Source: CAD feature listing. Evaluate the final solid. Frame: model axes, mm. Face numbers are marked on the shaded views. A direction names the side the tool comes from. Give positions to 0.01 mm unless a question says otherwise; leave off trailing zeros. Loops run counter-clockwise (first coordinate to the right, second up) from the corner with the lowest first, then second, coordinate; pieces in that order, holes last. Notation, with made-up numbers: M -25,39 L 30,39 A23 ccw 30,78 Z; hole C 64.25,-8.75 d1. An arc over 180 degrees is marked long. Answer in a Markdown table with one row per item.
```python
from build123d import *

# Parameters (mm, degrees)
BOSS_EXTRUDE1_DEPTH           = 12.7
SKETCH3_W                     = 9.525
SKETCH3_H                     = 3.683
BOSS_EXTRUDE2_DEPTH           = 1.2573
BOSS_EXTRUDE2_DRAFT           = 24.44
BOSS_EXTRUDE2_PROFILE_2_DEPTH = 1.2573
BOSS_EXTRUDE2_PROFILE_2_DRAFT = 24.44
BOSS_EXTRUDE2_PROFILE_3_DEPTH = 1.2573
BOSS_EXTRUDE2_PROFILE_3_DRAFT = 24.44
SKETCH2_W                     = 1.5875
SKETCH2_H                     = 4.191
BOSS_EXTRUDE3_DEPTH           = 5.3848
SKETCH4_W                     = 3.96875
SKETCH4_H                     = 4.191
BOSS_EXTRUDE4_DEPTH           = 3.175
CUT_EXTRUDE1_START            = -14.351
CUT_EXTRUDE1_DEPTH            = 14.351
FILLET1_R                     = 0.254


with BuildPart() as part:
    # Sketch1 → Boss-Extrude1 (new body)
    with BuildSketch(Plane.XY):
        with BuildLine():
            Line((3.554693097, 0.436578304), (13.826745412, 12.247578304))
            ThreePointArc((13.826745412, 12.247578304), (14.024174489, 13.607523715), (12.868461386, 14.351))
            Line((12.868461386, 14.351), (0, 14.351))
            Line((0, 14.351), (0, 0))
            Line((0, 0), (2.596409071, 0))
            ThreePointArc((2.596409071, 0), (3.122932786, 0.114286897), (3.554693097, 0.436578304))
        make_face()
    extrude(amount=BOSS_EXTRUDE1_DEPTH)


with BuildPart() as boss_extrude2_tool:
    # Sketch3 → Boss-Extrude2 (with draft: the straight prism first)
    with BuildSketch(Plane.ZY):
        with Locations((6.35, 7.1755)):
            Rectangle(SKETCH3_W, SKETCH3_H)
    extrude(amount=BOSS_EXTRUDE2_DEPTH)
    # Boss-Extrude2: the draft: its side faces are tilted about the plane it starts from
    boss_extrude2_sides = [boss_extrude2_tool.faces().sort_by_distance(p)[0] for p in [
        (-0.62865, 7.1755, 1.5875),
        (-0.62865, 5.334, 6.35),
        (-0.62865, 7.1755, 11.1125),
        (-0.62865, 9.017, 6.35),
    ]]
    draft(boss_extrude2_sides, Plane.ZY, BOSS_EXTRUDE2_DRAFT)


with BuildPart() as part_1:
    add(part.part)

    # Boss-Extrude2: add boss_extrude2_tool
    add(boss_extrude2_tool.part)


with BuildPart() as boss_extrude2_profile_2_tool:
    # Sketch3 → Boss-Extrude2 profile 2 (with draft: the straight prism first)
    with BuildSketch(Plane.ZY):
        with Locations((6.35, 12.5095)):
            Rectangle(SKETCH3_W, SKETCH3_H)
    extrude(amount=BOSS_EXTRUDE2_PROFILE_2_DEPTH)
    # Boss-Extrude2 profile 2: the draft: its side faces are tilted about the plane it starts from
    boss_extrude2_profile_2_sides = [boss_extrude2_profile_2_tool.faces().sort_by_distance(p)[0] for p in [
        (-0.62865, 12.5095, 1.5875),
        (-0.62865, 10.668, 6.35),
        (-0.62865, 12.5095, 11.1125),
        (-0.62865, 14.351, 6.35),
    ]]
    draft(boss_extrude2_profile_2_sides, Plane.ZY, BOSS_EXTRUDE2_PROFILE_2_DRAFT)


with BuildPart() as part_2:
    add(part_1.part)

    # Boss-Extrude2 profile 2: add boss_extrude2_profile_2_tool
    add(boss_extrude2_profile_2_tool.part)


with BuildPart() as boss_extrude2_profile_3_tool:
    # Sketch3 → Boss-Extrude2 profile 3 (with draft: the straight prism first)
    with BuildSketch(Plane.ZY):
        with Locations((6.35, 1.8415)):
            Rectangle(SKETCH3_W, SKETCH3_H)
    extrude(amount=BOSS_EXTRUDE2_PROFILE_3_DEPTH)
    # Boss-Extrude2 profile 3: the draft: its side faces are tilted about the plane it starts from
    boss_extrude2_profile_3_sides = [boss_extrude2_profile_3_tool.faces().sort_by_distance(p)[0] for p in [
        (-0.62865, 1.8415, 1.5875),
        (-0.62865, 0, 6.35),
        (-0.62865, 1.8415, 11.1125),
        (-0.62865, 3.683, 6.35),
    ]]
    draft(boss_extrude2_profile_3_sides, Plane.ZY, BOSS_EXTRUDE2_PROFILE_3_DRAFT)


with BuildPart() as part_3:
    add(part_2.part)

    # Boss-Extrude2 profile 3: add boss_extrude2_profile_3_tool
    add(boss_extrude2_profile_3_tool.part)

    # Sketch2 → Boss-Extrude3 (add)
    with BuildSketch(Plane.ZY):
        with Locations((0.79375, 12.2555)):
            Rectangle(SKETCH2_W, SKETCH2_H)
        with Locations((0.79375, 2.0955)):
            Rectangle(SKETCH2_W, SKETCH2_H)
        with Locations((11.90625, 2.0955)):
            Rectangle(SKETCH2_W, SKETCH2_H)
        with Locations((11.90625, 12.2555)):
            Rectangle(SKETCH2_W, SKETCH2_H)
    extrude(amount=BOSS_EXTRUDE3_DEPTH)

    # Sketch4 → Boss-Extrude4 (add)
    with BuildSketch(Plane.ZY.offset(5.3848)):
        with Locations((1.984375, 12.2555)):
            Rectangle(SKETCH4_W, SKETCH4_H)
        with Locations((10.715625, 12.2555)):
            Rectangle(SKETCH4_W, SKETCH4_H)
        with Locations((10.715625, 2.0955)):
            Rectangle(SKETCH4_W, SKETCH4_H)
        with Locations((1.984375, 2.0955)):
            Rectangle(SKETCH4_W, SKETCH4_H)
    extrude(amount=BOSS_EXTRUDE4_DEPTH)

    # Sketch5 → Cut-Extrude1 (cut)
    with BuildSketch(Plane.XZ.offset(CUT_EXTRUDE1_START)):
        Polygon((-5.3848, 3.96875), (-8.5598, 0), (-8.5598, 3.96875), align=None)
        Polygon((-8.5598, 12.7), (-8.5598, 8.73125), (-5.3848, 8.73125), align=None)
    extrude(amount=CUT_EXTRUDE1_DEPTH, mode=Mode.SUBTRACT)

    # Fillet1
    fillet1_edges = [part_3.edges().sort_by_distance(p)[0] for p in [
        (-8.5598, 12.2555, 0),
        (-8.5598, 2.0955, 12.7),
        (-8.5598, 12.2555, 12.7),
        (-8.5598, 2.0955, 0),
    ]]
    fillet(fillet1_edges, radius=FILLET1_R)


solid = part_3.part
```
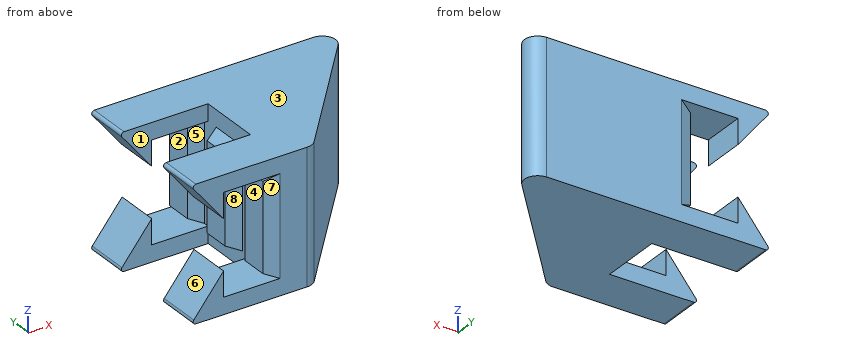
Q1. Contact query for flat-ended pins moving along their axis: pin 1 Ø1.3 at (y, z) = (1.5, 5) entering from -X; pin 2 Ø4 at (x, z) = (10, 3.5) entering from -Y; pin 3 Ø2 at (x, y) = (9, 4) entering from +Z; pin 4 Ø2 at (y, z) = (12.5, 4.5) entering from -X. Output: stop coordinate, or through.
Values follow:
| item | result |
|---|---|
| pin 1 | x = -1.26 |
| pin 2 | y = 5.55 |
| pin 3 | through |
| pin 4 | x = -5.76 |
Q2. Mould query, pull axis Z, two halves, no side actions, for the marked faces 1, 2 and 3. Classes: +Z half, -Z half, draft (parallel to the pull), parting line (faces both ways), or undercut.
Values follow:
| item | result |
|---|---|
| face 1 | draft |
| face 2 | undercut |
| face 3 | +Z half |
Q3. Section query D-D (y = 8). Output: boundary loops of the cut face in (x, z).
Values follow:
| item | result |
|---|---|
| outline | M -1.26,2.16 L 0,1.59 L 0,0 L 10.13,0 L 10.13,12.7 L 0,12.7 L 0,11.11 L -1.26,10.54 Z |
Q4. Reachability of the marked faces 4, 5, 6, 7 and 8 from +Z, -Z, +X, -X, +Y, -Y: full face, straight path, thin tool, end or side. Return the list, or none.
Values follow:
| item | result |
|---|---|
| face 4 | +Y, -Y |
| face 5 | none |
| face 6 | -X, +Y, -Y |
| face 7 | -Y |
| face 8 | +Z, -Z, -X |
Q5. Section query A-A (x = -2.75). Output: boundary loops of the cut face in (y, z).
Values follow:
| item | result |
|---|---|
| outline | M 0,0 L 4.19,0 L 4.19,1.59 L 0,1.59 Z; M 0,11.11 L 4.19,11.11 L 4.19,12.7 L 0,12.7 Z; M 10.16,0 L 14.35,0 L 14.35,1.59 L 10.16,1.59 Z; M 10.16,11.11 L 14.35,11.11 L 14.35,12.7 L 10.16,12.7 Z |
Q6. Section query B-B (z = 6.75). Output: boundary loops of the cut face in (x, y), plus the area to 3 significant figures.
Values follow:
| item | result |
|---|---|
| outline | M -1.26,0.57 L 0,0 L 2.6,0 A1.27 ccw 3.55,0.44 L 13.83,12.25 A1.27 ccw 12.87,14.35 L 0,14.35 L -1.26,13.78 L -1.26,11.24 L 0,10.67 L 0,9.02 L -1.26,8.45 L -1.26,5.91 L 0,5.33 L 0,3.68 L -1.26,3.11 Z |
| area | 145 mm^2 |
Q7. Section query C-C (z = 3.25). Output: boundary loops of the cut face in (x, y).
Values follow:
| item | result |
|---|---|
| outline | M -5.96,0 L -5.38,0 L -5.38,4.19 L -5.96,4.19 Z; M -5.96,10.16 L -5.38,10.16 L -5.38,14.35 L -5.96,14.35 Z; M -1.26,0.57 L 0,0 L 2.6,0 A1.27 ccw 3.55,0.44 L 13.83,12.25 A1.27 ccw 12.87,14.35 L 0,14.35 L -1.26,13.78 L -1.26,11.24 L 0,10.67 L 0,9.02 L -1.26,8.45 L -1.26,5.91 L 0,5.33 L 0,3.68 L -1.26,3.11 Z |
Q8. Ray query, probe 1 along Y at (x, z) = (-2.5, 1.5); probe 2 along Z at (x, y) = (-4, 13.75); probe 3 along Y at (x, z) = (-0.25, 6). Return the intervals inside material, ascending. Write a range as from..to.
Values follow:
| item | result |
|---|---|
| probe 1 | 0..4.19, 10.16..14.35 |
| probe 2 | 0..1.59, 11.11..12.7 |
| probe 3 | 0.11..3.57, 5.45..8.9, 10.78..14.24 |
